Build history of the part. All positions in model axes, mm. A direction names the side the tool comes from. Round coordinates to 2 decimals unless told otherwise and drop trailing zeros. Write each loop counter-clockwise with the first axis right and the second up, starting at its lowest first coordinate (ties: lowest second). Pieces come first, ordered by that corner, then holes. Notation, with made-up numbers: (-3.75, 6) - (31.25, 6) arc R23 ccw to (31.25, 15) - close; hole circle Ø1 at (-21.5, 8.5). An arc over 180 degrees is marked (long way). Answer as a JSON object with one key per item and string values. Group by question number.
Item 1: Slice it at A-A, the plane y = 5. List the corners of the cut face in (x, z).
Item 2: Which spindle directions (+Z, -Z, +X, -X, +Y, -Y) get a long thin tool onto all of the face, cutting with end or side? Do faces 5 (the cylindrical face through (-32.45, 20.55, 2.58)), 6 (the flat face through (-73.31, 5, 6)), 7 (the flat face through (-13, -5, 3)). Say none if no direction does.
Item 3: Probe line 1 (Y direction, x = -12, z = 7); line 2 (Y direction, x = -30.5, z = 6.75); line 3 (X direction, y = 3.5, z = 6.75). List the from-to ranges inside material, lowest first. Write a range as from..to.
Item 4: Slice it at B-B, the plane x = -12. List the corners of the cut face in (y, z).
Item 5: Slice it at D-D, the plane z = -1. List the corners of the cut face in (x, y).
Item 6: Flat gauge pins, fed straight in: pin 1 (3.5 mm diameter, centred on x = -8.5, z = 3, fed in from -Y); pin 2 (4 mm diameter, centred on x = -30, z = 0.5, fed in from +Y); pin 3 (1.5 mm diameter, centred on x = -75, z = 2.5, fed in from -Y). Where does each tip first touch, or does it go through?
Item 7: Two-plate mould, pull along Y, no slides. Class faces 1 (the flat face through (-14, 12.16, 4)), 2 (the cylindrical face through (-74.599, 19.166, 2.577)), 3 (the flat face through (2, -2, 11)), 4 (the cylindrical face through (3.289, -3.196, 2.577)): +Y half, -Y half, draft (parallel to the pull), parting line (faces both ways), or undercut.
from build123d import *

# Parameters (mm, degrees)
SKETCH3_R                = 1
BOSS_EXTRUDE2_DEPTH      = 8
BOSS_EXTRUDE2_DEPTH_BACK = 3
BOSS_EXTRUDE3_DEPTH      = 3
SKETCH7_R                = 1
BOSS_EXTRUDE4_DEPTH      = 3
BOSS_EXTRUDE4_DEPTH_BACK = 11
SKETCH9_W                = 5
SKETCH9_H                = 19.78
CUT_EXTRUDE2_DEPTH       = 10


with BuildPart() as part:
    # Sketch3 → Boss-Extrude2 (new, two sides)
    with BuildSketch(Plane.XY) as boss_extrude2_sk:
        with BuildLine():
            Line((-70.31, 20.97), (-34.65285742, 20.97))
            ThreePointArc((-34.65285742, 20.97), (-32.418966384, 20.53863815), (-30.506280473, 19.306576947))
            Line((-30.506280473, 19.306576947), (-26.169703525, 15.16))
            Line((-26.169703525, 15.16), (-1, 15.16))
            ThreePointArc((-1, 15.16), (3.242640687, 13.402640687), (5, 9.16))
            Line((5, 9.16), (5, 1))
            ThreePointArc((5, 1), (3.242640687, -3.242640687), (-1, -5))
            Line((-1, -5), (-26.169703525, -5))
            Line((-26.169703525, -5), (-30.506280473, -9.146576947))
            ThreePointArc((-30.506280473, -9.146576947), (-32.418966384, -10.37863815), (-34.65285742, -10.81))
            Line((-34.65285742, -10.81), (-70.31, -10.81))
            ThreePointArc((-70.31, -10.81), (-74.552640687, -9.052640687), (-76.31, -4.81))
            Line((-76.31, -4.81), (-76.31, 14.97))
            ThreePointArc((-76.31, 14.97), (-74.552640687, 19.212640687), (-70.31, 20.97))
        make_face()
        with Locations((-73.31, 17.97)):
            Circle(SKETCH3_R, mode=Mode.SUBTRACT)
        with Locations((-73.31, -7.81)):
            Circle(SKETCH3_R, mode=Mode.SUBTRACT)
        with Locations((2, -2)):
            Circle(SKETCH3_R, mode=Mode.SUBTRACT)
        with Locations((2, 12.16)):
            Circle(SKETCH3_R, mode=Mode.SUBTRACT)
        with BuildLine():
            Line((-70.31, 17.97), (-34.65285742, 17.97))
            ThreePointArc((-34.65285742, 17.97), (-33.535911902, 17.754319075), (-32.579568946, 17.138288474))
            Line((-32.579568946, 17.138288474), (-28.242991999, 12.991711526))
            ThreePointArc((-28.242991999, 12.991711526), (-27.286649043, 12.375680925), (-26.169703525, 12.16))
            Line((-26.169703525, 12.16), (-1, 12.16))
            ThreePointArc((-1, 12.16), (1.121320344, 11.281320344), (2, 9.16))
            Line((2, 9.16), (2, 1))
            ThreePointArc((2, 1), (1.121320344, -1.121320344), (-1, -2))
            Line((-1, -2), (-26.169703525, -2))
            ThreePointArc((-26.169703525, -2), (-27.286649043, -2.215680925), (-28.242991999, -2.831711526))
            Line((-28.242991999, -2.831711526), (-32.579568946, -6.978288474))
            ThreePointArc((-32.579568946, -6.978288474), (-33.535911902, -7.594319075), (-34.65285742, -7.81))
            Line((-34.65285742, -7.81), (-70.31, -7.81))
            ThreePointArc((-70.31, -7.81), (-72.431320344, -6.931320344), (-73.31, -4.81))
            Line((-73.31, -4.81), (-73.31, 14.97))
            ThreePointArc((-73.31, 14.97), (-72.431320344, 17.091320344), (-70.31, 17.97))
        make_face(mode=Mode.SUBTRACT)
    extrude(amount=BOSS_EXTRUDE2_DEPTH)
    extrude(boss_extrude2_sk.sketch, amount=-BOSS_EXTRUDE2_DEPTH_BACK)

    # Sketch5 → Boss-Extrude3 (add)
    with BuildSketch(Plane(origin=(0, 0, -3), x_dir=(-1, 0, 0), z_dir=(0, 0, -1))):
        with BuildLine():
            Line((73.31, 14.97), (73.31, -4.81))
            ThreePointArc((73.31, -4.81), (72.431320344, -6.931320344), (70.31, -7.81))
            Line((70.31, -7.81), (34.65285742, -7.81))
            ThreePointArc((34.65285742, -7.81), (33.535911902, -7.594319075), (32.579568946, -6.978288474))
            Line((32.579568946, -6.978288474), (28.242991999, -2.831711526))
            ThreePointArc((28.242991999, -2.831711526), (27.286649043, -2.215680925), (26.169703525, -2))
            Line((26.169703525, -2), (1, -2))
            ThreePointArc((1, -2), (-1.121320344, -1.121320344), (-2, 1))
            Line((-2, 1), (-2, 9.16))
            ThreePointArc((-2, 9.16), (-1.121320344, 11.281320344), (1, 12.16))
            Line((1, 12.16), (26.169703525, 12.16))
            ThreePointArc((26.169703525, 12.16), (27.286649043, 12.375680925), (28.242991999, 12.991711526))
            Line((28.242991999, 12.991711526), (32.579568946, 17.138288474))
            ThreePointArc((32.579568946, 17.138288474), (33.535911902, 17.754319075), (34.65285742, 17.97))
            Line((34.65285742, 17.97), (70.31, 17.97))
            ThreePointArc((70.31, 17.97), (72.431320344, 17.091320344), (73.31, 14.97))
        make_face()
    extrude(amount=-BOSS_EXTRUDE3_DEPTH)

    # Sketch7 → Boss-Extrude4 (add, two sides)
    with BuildSketch(Plane.XY.offset(8)) as boss_extrude4_sk:
        with Locations((-73.31, 17.97)):
            Circle(SKETCH7_R)
        with Locations((2, -2)):
            Circle(SKETCH7_R)
        with Locations((2, 12.16)):
            Circle(SKETCH7_R)
        with Locations((-73.31, -7.81)):
            Circle(SKETCH7_R)
    extrude(amount=BOSS_EXTRUDE4_DEPTH)
    extrude(boss_extrude4_sk.sketch, amount=-BOSS_EXTRUDE4_DEPTH_BACK)

    # Sketch9 → Cut-Extrude2 (cut)
    with BuildSketch(Plane.ZY.offset(76.31)):
        with Locations((2.5, 5.08)):
            Rectangle(SKETCH9_W, SKETCH9_H)
    extrude(amount=-CUT_EXTRUDE2_DEPTH, mode=Mode.SUBTRACT)


solid = part.part
Geometry says:
{
 "1": {"outline": "(-76.31, -3) - (5, -3) - (5, 8) - (2, 8) - (2, 0) - (-76.31, 0) - close; (-76.31, 5) - (-73.31, 5) - (-73.31, 8) - (-76.31, 8) - close"},
 "2": {"face 5": "+Z, -Z, +X, +Y", "face 6": "+Z", "face 7": "+Z, -Z, +X, -Y"},
 "3": {"line 1": "y = -5..-2, 12.16..15.16", "line 2": "y = -9.14..-4.99, 15.15..19.3", "line 3": "x = -76.31..-73.31, 2..5"},
 "4": {"outline": "(-5, -3) - (15.16, -3) - (15.16, 8) - (12.16, 8) - (12.16, 0) - (-2, 0) - (-2, 8) - (-5, 8) - close"},
 "5": {"outline": "(-76.31, -4.81) arc R6 ccw to (-70.31, -10.81) - (-34.65, -10.81) arc R6 ccw to (-30.51, -9.15) - (-26.17, -5) - (-1, -5) arc R6 ccw to (5, 1) - (5, 9.16) arc R6 ccw to (-1, 15.16) - (-26.17, 15.16) - (-30.51, 19.31) arc R6 ccw to (-34.65, 20.97) - (-70.31, 20.97) arc R6 ccw to (-76.31, 14.97) - close"},
 "6": {"pin 1": "stops at y = -5", "pin 2": "stops at y = 20.35", "pin 3": "stops at y = -9.34"},
 "7": {"face 1": "undercut", "face 2": "+Y half", "face 3": "draft", "face 4": "-Y half"}
}
